For this review, take the finished solid that the model builds, in its own axes (mm). A direction names the side the tool comes from. Round coordinates to 2 decimals unless told otherwise and drop trailing zeros. Use a Markdown table: item, result. Add a question column.
1) Draft analysis for pull direction X (two halves, no side actions). For faces 1 (the face through (-0.38, 209.64, 20.99)), 2 (the face through (-20.99, 209.64, 0.38)), 3 (the face through (-26.005, 77.267, -24.61)), state which applies: pulls with the +X half, pulls with the -X half, needs draft (parallel to the pull), parting line crosses it, or undercut.
2) Wall thickness on line 1 along Z through (x, y) = (0, 59) (3 decimals); line 2 along Z through (x, y) = (23, 46): over which ranges is each line inside the solid? List them lowest first. Write a range as [from, to].
3) Machinability: for faces 4 (the face through (-7.559, 194.33, -5.796)), 5 (the face through (24.18, 77.27, -26.14)), 6 (the face through (-0.38, 209.64, -20.99)), which of the approach directions +Z, -Z, +X, -X, +Y, -Y give a long, thin tool a straight path to every point of the face, cutting with its end or side? Answer none if there is none.
4) Clearance check with flat-ended pins moving along their axes: P1, Ø4, axis at x = -23.622, z = -23.622, coming from the +Y side; P2, Ø6, axis at x = 23.622, z = -23.622, coming from the +Y side; P3, Ø12, axis at x = -3, z = 1.5, coming from the +Y side; P4, Ø10, axis at x = 3, z = -7, coming from the -Y side. State where each tip first meets the part, or that it passes through.
5) Consider section A-A (y = 87). Give the number of separate pieces and of enclosed holes in the cut face, plus the area to 3 significant figures.
```python
from build123d import *

# Parameters (mm, degrees)
SKETCH1_W                            = 54.864
SKETCH1_H                            = 54.864
BOSS_EXTRUDE2_DEPTH                  = 215.9
F_3_4_0_75_DIAMETER_HOLE1_D          = 19.05
F_3_4_0_75_DIAMETER_HOLE1_DEPTH      = 152.4
F_3_4_0_75_DIAMETER_HOLE1_TIP        = 5.723197396
F_13_64_0_20313_DIAMETER_HOLE1_D     = 5.159502
F_13_64_0_20313_DIAMETER_HOLE1_DEPTH = 152.4
F_13_64_0_20313_DIAMETER_HOLE1_TIP   = 1.550070783
F_3_4_0_75_DIAMETER_HOLE2_D          = 19.05
F_3_4_0_75_DIAMETER_HOLE2_DEPTH      = 42.545
F_3_4_0_75_DIAMETER_HOLE2_TIP        = 5.723197396
CHAMFER1_SIZE                        = 12.7


with BuildPart() as part:
    # Sketch1 → Boss-Extrude2 (new body)
    with BuildSketch(Plane(origin=(0, 0, 0), x_dir=(1, 0, 0), z_dir=(0, 1, 0))):
        Rectangle(SKETCH1_W, SKETCH1_H)
    extrude(amount=BOSS_EXTRUDE2_DEPTH)

    # 3/4 (0.75) Diameter Hole1
    with Locations(Plane.XZ):
        with Locations((0, 0)):
            Hole(F_3_4_0_75_DIAMETER_HOLE1_D / 2, depth=F_3_4_0_75_DIAMETER_HOLE1_DEPTH)
            with Locations((0, 0, -(F_3_4_0_75_DIAMETER_HOLE1_DEPTH + F_3_4_0_75_DIAMETER_HOLE1_TIP / 2))):  # 118° drill point
                Cone(0, F_3_4_0_75_DIAMETER_HOLE1_D / 2, F_3_4_0_75_DIAMETER_HOLE1_TIP, mode=Mode.SUBTRACT)

    # 13/64 (0.20313) Diameter Hole1
    with Locations(Plane.XZ):
        with Locations((-23.622, 23.622), (23.622, 23.622), (23.622, -23.622), (-23.622, -23.622)):
            Hole(F_13_64_0_20313_DIAMETER_HOLE1_D / 2, depth=F_13_64_0_20313_DIAMETER_HOLE1_DEPTH)
            with Locations((0, 0, -(F_13_64_0_20313_DIAMETER_HOLE1_DEPTH + F_13_64_0_20313_DIAMETER_HOLE1_TIP / 2))):  # 118° drill point
                Cone(0, F_13_64_0_20313_DIAMETER_HOLE1_D / 2, F_13_64_0_20313_DIAMETER_HOLE1_TIP, mode=Mode.SUBTRACT)

    # 3/4 (0.75) Diameter Hole2
    with Locations(Plane(origin=(0, 215.9, 0), x_dir=(-1, 0, 0), z_dir=(0, 1, 0))):
        with Locations((0, 0)):
            Hole(F_3_4_0_75_DIAMETER_HOLE2_D / 2, depth=F_3_4_0_75_DIAMETER_HOLE2_DEPTH)
            with Locations((0, 0, -(F_3_4_0_75_DIAMETER_HOLE2_DEPTH + F_3_4_0_75_DIAMETER_HOLE2_TIP / 2))):  # 118° drill point
                Cone(0, F_3_4_0_75_DIAMETER_HOLE2_D / 2, F_3_4_0_75_DIAMETER_HOLE2_TIP, mode=Mode.SUBTRACT)

    # Chamfer1
    chamfer1_edges = [part.edges().sort_by_distance(p)[0] for p in [
        (0, 215.9, 27.432),
        (-27.432, 215.9, 0),
        (0, 215.9, -27.432),
        (27.432, 215.9, 0),
    ]]
    chamfer(chamfer1_edges, length=CHAMFER1_SIZE)


solid = part.part
```
Results list:
| question | item | result |
|---|---|---|
| 1 | face 1 | needs draft |
| 1 | face 2 | pulls with the -X half |
| 1 | face 3 | undercut |
| 2 | line 1 | [-27.432, -9.525], [9.525, 27.432] |
| 2 | line 2 | [-27.43, -26.13], [-21.12, 21.12], [26.13, 27.43] |
| 3 | face 4 | +Y |
| 3 | face 5 | -Y |
| 3 | face 6 | -Z, +X, -X, +Y |
| 4 | P1 | y = 208.42 |
| 4 | P2 | y = 209.13 |
| 4 | P3 | y = 173.25 |
| 4 | P4 | y = 0 |
| 5 | separate pieces | 1 |
| 5 | enclosed holes | 5 |
| 5 | area | 2,640 mm2 |
